Build history of the part. All positions in model axes, mm. Face numbers are marked on the shaded views. A direction names the side the tool comes from. Round coordinates to 2 decimals unless told otherwise and drop trailing zeros. Loops run counter-clockwise (first coordinate to the right, second up) from the corner with the lowest first, then second, coordinate; pieces in that order, holes last.
from build123d import *

# Parameters (mm, degrees)
SKETCH1_W           = 46.5
SKETCH1_H           = 34.5
BOSS_EXTRUDE1_DEPTH = 4
SKETCH2_W           = 46.5
SKETCH2_H           = 2.95
BOSS_EXTRUDE2_DEPTH = 6.5
SKETCH3_R           = 1.25
CUT_EXTRUDE1_DEPTH  = 35.5
CUT_EXTRUDE8_DEPTH  = 35.5
SKETCH5_R           = 0.725
CUT_EXTRUDE3_DEPTH  = 11.25
SKETCH21_W          = 12.4
SKETCH21_H          = 8.2
CUT_EXTRUDE11_DEPTH = 11.25
BOSS_EXTRUDE3_DEPTH = 0.1
BOSS_EXTRUDE4_DEPTH = 0.1
SKETCH17_W          = 10.25
SKETCH17_H          = 34.5
BOSS_EXTRUDE6_DEPTH = 1.9
SKETCH18_W          = 10.25
SKETCH18_H          = 34.5
BOSS_EXTRUDE7_DEPTH = 1.9
CUT_EXTRUDE10_DEPTH = 51.5
CHAMFER1_SIZE       = 2
FILLET2_R           = 1
CUT_EXTRUDE12_DEPTH = 2


with BuildPart() as part:
    # Sketch1 → Boss-Extrude1 (new body)
    with BuildSketch(Plane.XY):
        Rectangle(SKETCH1_W, SKETCH1_H)
    extrude(amount=BOSS_EXTRUDE1_DEPTH)

    # Sketch2 → Boss-Extrude2 (add)
    with BuildSketch(Plane.XY.offset(4)):
        with Locations((0, 15.775)):
            Rectangle(SKETCH2_W, SKETCH2_H)
        with Locations((0, -15.775)):
            Rectangle(SKETCH2_W, SKETCH2_H)
    extrude(amount=BOSS_EXTRUDE2_DEPTH)

    # Sketch3 → Cut-Extrude1 (cut, through all)
    with BuildSketch(Plane(origin=(0, 17.25, 0), x_dir=(1, 0, 0), z_dir=(0, 1, 0))):
        with Locations((-20, -7.25)):
            Circle(SKETCH3_R)
        with Locations((20, -7.25)):
            Circle(SKETCH3_R)
    extrude(amount=-CUT_EXTRUDE1_DEPTH, mode=Mode.SUBTRACT)

    # Sketch11 → Cut-Extrude8 (cut, through all)
    with BuildSketch(Plane(origin=(0, 17.25, 0), x_dir=(1, 0, 0), z_dir=(0, 1, 0))):
        with BuildLine():
            Line((-17, -7.25), (-17, -4))
            Line((-17, -4), (17, -4))
            Line((17, -4), (17, -7.25))
            ThreePointArc((17, -7.25), (17.878679656, -9.371320344), (20, -10.25))
            Line((20, -10.25), (23.25, -10.25))
            Line((23.25, -10.25), (23.25, -10.5))
            Line((23.25, -10.5), (-23.25, -10.5))
            Line((-23.25, -10.5), (-23.25, -10.25))
            Line((-23.25, -10.25), (-20, -10.25))
            ThreePointArc((-20, -10.25), (-17.878679656, -9.371320344), (-17, -7.25))
        make_face()
    extrude(amount=-CUT_EXTRUDE8_DEPTH, mode=Mode.SUBTRACT)

    # Sketch5 → Cut-Extrude3 (cut, through all)
    with BuildSketch(Plane(origin=(0, 0, 0), x_dir=(-1, 0, 0), z_dir=(0, 0, -1))):
        with Locations((8, 6)):
            Circle(SKETCH5_R)
        with Locations((8, -6)):
            Circle(SKETCH5_R)
        with Locations((-16, -6)):
            Circle(SKETCH5_R)
        with Locations((-16, 6)):
            Circle(SKETCH5_R)
    extrude(amount=-CUT_EXTRUDE3_DEPTH, mode=Mode.SUBTRACT)

    # Sketch21 → Cut-Extrude11 (cut, through all)
    with BuildSketch(Plane(origin=(0, 0, 0), x_dir=(-1, 0, 0), z_dir=(0, 0, -1))):
        with Locations((-2.05, -13.6)):
            Rectangle(SKETCH21_W, SKETCH21_H)
    extrude(amount=-CUT_EXTRUDE11_DEPTH, mode=Mode.SUBTRACT)

    # Sketch14 → Boss-Extrude3 (add)
    with BuildSketch(Plane.ZY.offset(23.25)):
        Polygon((10.25, 17.25), (0, 17.25), (0, -17.25), (10.25, -17.25), (10.25, -14.3), (4, -14.3), (4, 14.3), (10.25, 14.3), align=None)
    extrude(amount=BOSS_EXTRUDE3_DEPTH)

    # Sketch15 → Boss-Extrude4 (add)
    with BuildSketch(Plane(origin=(23.25, 0, 0), x_dir=(0, 0, -1), z_dir=(1, 0, 0))):
        Polygon((-10.25, -17.25), (0, -17.25), (0, 17.25), (-10.25, 17.25), (-10.25, 14.3), (-4, 14.3), (-4, -14.3), (-10.25, -14.3), align=None)
    extrude(amount=BOSS_EXTRUDE4_DEPTH)

    # Sketch17 → Boss-Extrude6 (add)
    with BuildSketch(Plane.ZY.offset(23.35)):
        with Locations((5.125, 0)):
            Rectangle(SKETCH17_W, SKETCH17_H)
    extrude(amount=BOSS_EXTRUDE6_DEPTH)

    # Sketch18 → Boss-Extrude7 (add)
    with BuildSketch(Plane(origin=(23.35, 0, 0), x_dir=(0, 0, -1), z_dir=(1, 0, 0))):
        with Locations((-5.125, 0)):
            Rectangle(SKETCH18_W, SKETCH18_H)
    extrude(amount=BOSS_EXTRUDE7_DEPTH)

    # Sketch19 → Cut-Extrude10 (cut, through all)
    with BuildSketch(Plane.ZY.offset(25.25)):
        Polygon((10.25, 12.3), (7, 12.3), (4, 9.3), (4, -9.3), (7, -12.3), (10.25, -12.3), align=None)
    extrude(amount=-CUT_EXTRUDE10_DEPTH, mode=Mode.SUBTRACT)

    # Chamfer1
    chamfer1_edges = [part.edges().sort_by_distance(p)[0] for p in [
        (16.75, -17.25, 0),
        (-25.25, 0, 0),
        (-25.25, -17.25, 5.125),
        (-25.25, 17.25, 5.125),
        (25.25, 0, 0),
        (25.25, 17.25, 5.125),
        (25.25, -17.25, 5.125),
        (-24.3, 12.3, 10.25),
        (-24.3, -12.3, 10.25),
        (24.3, 12.3, 10.25),
        (24.3, -12.3, 10.25),
        (0, 17.25, 0),
        (-14.7, -17.25, 0),
    ]]
    chamfer(chamfer1_edges, length=CHAMFER1_SIZE)

    # Fillet2
    fillet2_edges = [part.edges().sort_by_distance(p)[0] for p in [
        (-4.15, -9.5, 2),
        (8.25, -9.5, 2),
    ]]
    fillet(fillet2_edges, radius=FILLET2_R)

    # Sketch22 → Cut-Extrude12 (cut)
    with BuildSketch(Plane.XY.offset(4)):
        Polygon((-7.133974596, 4.5), (-6.267949192, 6), (-7.133974596, 7.5), (-8.866025404, 7.5), (-9.732050808, 6), (-8.866025404, 4.5), align=None)
        Polygon((-7.133974596, -7.5), (-6.267949192, -6), (-7.133974596, -4.5), (-8.866025404, -4.5), (-9.732050808, -6), (-8.866025404, -7.5), align=None)
        Polygon((16.866025404, -7.5), (17.732050808, -6), (16.866025404, -4.5), (15.133974596, -4.5), (14.267949192, -6), (15.133974596, -7.5), align=None)
        Polygon((16.866025404, 4.5), (17.732050808, 6), (16.866025404, 7.5), (15.133974596, 7.5), (14.267949192, 6), (15.133974596, 4.5), align=None)
    extrude(amount=-CUT_EXTRUDE12_DEPTH, mode=Mode.SUBTRACT)


solid = part.part
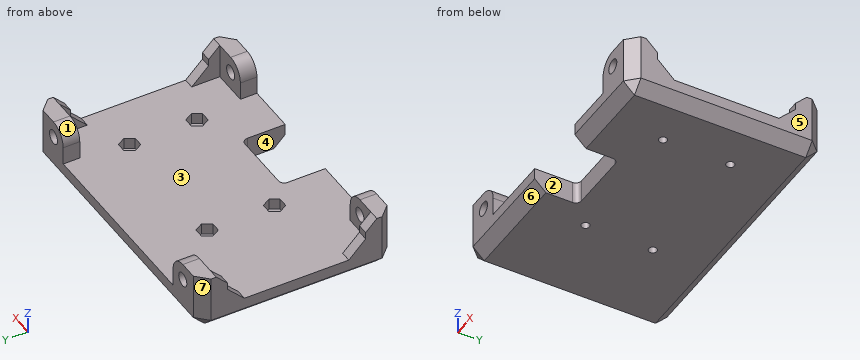
(1) Slice it at C-C on x = -2.5. List the corners of the cut face in (y, z).
Responses:
outline: (-9.5, 0) - (15.25, 0) - (17.25, 2) - (17.25, 4) - (-9.5, 4) - close
(2) Slice it at B-B on z = 9. List the corners of the cut face in (x, y), plus the area to 3 significant figures.
Responses:
outline: (-25.25, -15.25) - (-23.25, -17.25) - (-17.56, -17.25) - (-17.56, -14.3) - (-23.35, -14.3) - (-23.35, -13.05) - (-25.25, -13.05) - close; (-25.25, 13.05) - (-23.35, 13.05) - (-23.35, 14.3) - (-17.56, 14.3) - (-17.56, 17.25) - (-23.25, 17.25) - (-25.25, 15.25) - close; (17.56, -17.25) - (23.25, -17.25) - (25.25, -15.25) - (25.25, -13.05) - (23.35, -13.05) - (23.35, -14.3) - (17.56, -14.3) - close; (17.56, 14.3) - (23.35, 14.3) - (23.35, 13.05) - (25.25, 13.05) - (25.25, 15.25) - (23.25, 17.25) - (17.56, 17.25) - close
area: 92.2 mm2
(3) Slice it at A-A on x = -8. List the corners of the cut face in (y, z) (3 decimals).
Responses:
outline: (-17.25, 2) - (-15.25, 0) - (-6.725, 0) - (-6.725, 2) - (-7.5, 2) - (-7.5, 4) - (-17.25, 4) - close; (-5.275, 0) - (5.275, 0) - (5.275, 2) - (4.5, 2) - (4.5, 4) - (-4.5, 4) - (-4.5, 2) - (-5.275, 2) - close; (6.725, 0) - (15.25, 0) - (17.25, 2) - (17.25, 4) - (7.5, 4) - (7.5, 2) - (6.725, 2) - close
(4) Which spindle directions (+Z, -Z, +X, -X, +Y, -Y) get a long thin tool onto all of the face, cutting with end or side? Do the marked faces 1, 2 and 3. Say none if no direction does.
Responses:
face 1: +Z, +Y, -Y
face 2: +Z, -Z, -Y
face 3: +Z
(5) Probe line 1 (X direction, y = -14.95, z = 7.25); line 2 (Y direction, x = -7.5, z = 2.25); line 3 (X direction, y = 15.75, z = 7.25). List the from-to ranges inside material, lowest first.
Responses:
line 1: x = -25.25 to -21.25, -18.75 to -17, 17 to 18.75, 21.25 to 25.25
line 2: y = -17.25 to -7.5, -4.5 to 4.5, 7.5 to 17.25
line 3: x = -24.75 to -21.25, -18.75 to -17, 17 to 18.75, 21.25 to 24.75
(6) Pin check, flat tips, straight feed: P1, Ø0.9, axis at y = 16, z = 6, coming from the -X side; P2, Ø5, axis at x = 0.5, y = 7, coming from the +Z side; P3, Ø1.9, axis at x = 19.5, z = 6.5, coming from the -Y side. Stop position of each tip, or through.
Responses:
P1: stops at x = -24.95
P2: stops at z = 4
P3: stops at y = -17.25
(7) Pull direction X, two halves, no side cores. Call the marked faces 4, 5, 6 and 7: +X half, -X half, draft (parallel to the pull), parting line (faces both ways), or undercut.
Responses:
face 4: undercut
face 5: +X half
face 6: draft
face 7: -X half
